The model under review builds one solid part; all positions refer to its coordinate system, in mm. A direction names the side the tool comes from. Round coordinates to 2 decimals unless told otherwise and drop trailing zeros. Write each loop counter-clockwise with the first axis right and the second up, starting at its lowest first coordinate (ties: lowest second). Pieces come first, ordered by that corner, then holes. Notation, with made-up numbers: (46, -34.5) -> (51, -34.5) arc R26 cw to (51, 2.5) -> close; hole circle Ø1 at (-27, -32.75). An arc over 180 degrees is marked (long way). Return JSON: item names as keys, results as strings. Group by question number.
1. Take a section at C-C, the plane z = 0.5. Write out the cut boundary in (x, y), then the cut area to 3 significant figures.
2. For line 1 along X through (y, z) = (-0.75, -2.25); line 2 along Z through (x, y) = (-3, -1.05); line 3 along X through (y, z) = (-0.4, 4.5), list the stretches that pass through material, from the lowest coordinate up. Write a range as from..to.
3. Take a section at D-D, the plane x = -2.25. Write out the cut boundary in (y, z), then the cut area to 3 significant figures.
4. Mouldability with a two-part tool opening along Z and no side actions: class faces 1 (the flat face through (-0.1, -2, -1.6)), 2 (the cylindrical face through (-5.79, -0.99, 0.75)), 3 (the cylindrical face through (-1.63, -0.99, -7.32)) as pulls with the +Z half, pulls with the -Z half, needs draft (parallel to the pull), parting line crosses it, or undercut.
5. Tool access review of faces 4 (the flat face through (-4.144, -0.986, -1.81)), 5 (the flat face through (-0.1, 0, -1.6)): name each direction out of +Z, -Z, +X, -X, +Y, -Y from which nothing blocks a thin tool from reaching the whole face with its end or side.
6. Take a section at B-B, the plane x = -0.5. Write out the cut boundary in (y, z).
7. Take a section at A-A, the plane y = -1.2. Write out the cut boundary in (x, z) (1 decimal), then the cut area to 3 significant figures.
from build123d import *

# Parameters (mm, degrees)
F1_DEPTH = 2


# Not quite as in the source:
# - ends of sketch curves that miss each other by under 0.0002 mm in the source are joined


with BuildPart() as f1:
    # F0 (on Front) → F1 (new body)
    with BuildSketch(Plane.XZ):
        with BuildLine():
            ThreePointArc((-7.5, 0), (0, -7.5), (7.5, 0))
            ThreePointArc((7.5, 0), (0, 7.5), (-7.5, 0))
        make_face()
        with BuildLine():
            ThreePointArc((-9.252e-06, -5.837642026), (-0.8154481123, -5.781304427), (-1.6149720231, -5.6113751006))
            Line((-1.6149720231, -5.6113751006), (0, -2.0297722424))
            Line((0, -2.0297722424), (1.6130763481, -5.6119564271))
            ThreePointArc((1.6130763481, -5.6119564271), (0.8143893667, -5.7809478456), (-9.252e-06, -5.837642026))
        make_face(mode=Mode.SUBTRACT)
        with BuildLine():
            ThreePointArc((-5.8376432623, 4.535e-07), (-5.7885795806, 0.7619262356), (-5.6402209677, 1.5108774116))
            Line((-5.6402209677, 1.5108774116), (-2.6057938378, -5.2253115461))
            ThreePointArc((-2.6057938378, -5.2253115461), (-4.9642649621, -3.0719201723), (-5.8376432623, 4.535e-07))
        make_face(mode=Mode.SUBTRACT)
        with BuildLine():
            ThreePointArc((5.8375074432, 8.164e-07), (4.9638082552, -3.0717207498), (2.6056583249, -5.2253113695))
            Line((2.6056583249, -5.2253113695), (5.6435948014, 1.498042557))
            ThreePointArc((5.6435948014, 1.498042557), (5.7887533107, 0.7552604254), (5.8375074432, 8.164e-07))
        make_face(mode=Mode.SUBTRACT)
        with BuildLine():
            Line((0, 1.9682461262), (-1.6421023797, 5.6034935248))
            ThreePointArc((-1.6421023797, 5.6034935248), (-0.8294183969, 5.7791792496), (-8.9799e-06, 5.8374974962))
            ThreePointArc((-8.9799e-06, 5.8374974962), (0.8283723862, 5.7788128003), (1.6402065238, 5.6039289974))
            Line((1.6402065238, 5.6039289974), (0, 1.9682461262))
        make_face(mode=Mode.SUBTRACT)
        with BuildLine():
            Line((0.990821727, 0.1571487487), (3.1334508081, 4.9261166556))
            ThreePointArc((3.1334508081, 4.9261166556), (3.9933572695, 4.2579147754), (4.7150061526, 3.4423429304))
            Line((4.7150061526, 3.4423429304), (2.0229239131, -2.5149786417))
            Line((2.0229239131, -2.5149786417), (0.9841275984, -0.2051414777))
            Line((0.9841275984, -0.2051414777), (-0.9841094572, -0.2051414777))
            Line((-0.9841094572, -0.2051414777), (-2.0228967012, -2.5149786417))
            Line((-2.0228967012, -2.5149786417), (-4.7110881859, 3.447911577))
            ThreePointArc((-4.7110881859, 3.447911577), (-3.9911114988, 4.2602728506), (-3.1337140349, 4.925981317))
            Line((-3.1337140349, 4.925981317), (-0.9841094572, 0.1571487487))
            Line((-0.9841094572, 0.1571487487), (0.990821727, 0.1571487487))
        make_face(mode=Mode.SUBTRACT)
    extrude(amount=F1_DEPTH)


solid = f1.part
Output:
{
 "1": {"outline": "(-7.48, -2) -> (-5.82, -2) -> (-5.82, 0) -> (-7.48, 0) -> close; (-5.18, -2) -> (-3.38, -2) -> (-3.38, 0) -> (-5.18, 0) -> close; (-1.14, -2) -> (1.14, -2) -> (1.14, 0) -> (-1.14, 0) -> close; (3.39, -2) -> (5.19, -2) -> (5.19, 0) -> (3.39, 0) -> close; (5.82, -2) -> (7.48, -2) -> (7.48, 0) -> (5.82, 0) -> close", "area": "18.5 mm^2"},
 "2": {"line 1": "x = -7.15..-5.39, -3.95..-2.14, -1.9..-0.1, 0.1..1.9, 2.14..3.95, 5.39..7.15", "line 2": "z = -6.87..-5.01, -4.35..-0.35, 4.63..6.87", "line 3": "x = -6..-3.72, -2.94..-1.14, 1.14..2.94, 3.72..6"},
 "3": {"outline": "(-2, -7.15) -> (0, -7.15) -> (0, -2.01) -> (-2, -2.01) -> close; (-2, 2.97) -> (0, 2.97) -> (0, 7.15) -> (-2, 7.15) -> close", "area": "18.7 mm^2"},
 "4": {"face 1": "needs draft", "face 2": "undercut", "face 3": "parting line crosses it"},
 "5": {"face 4": "+Y, -Y", "face 5": "+Z, -Z, +X, -X, +Y"},
 "6": {"outline": "(-2, -7.48) -> (0, -7.48) -> (0, -5.82) -> (-2, -5.82) -> close; (-2, -3.14) -> (0, -3.14) -> (0, -0.21) -> (-2, -0.21) -> close; (-2, 0.16) -> (0, 0.16) -> (0, 3.08) -> (-2, 3.08) -> close; (-2, 5.82) -> (0, 5.82) -> (0, 7.48) -> (-2, 7.48) -> close"},
 "7": {"outline": "circle Ø15 at (0, 0); hole (-5.8, 0) arc R5.8 ccw to (-2.6, -5.2) -> (-5.6, 1.5) arc R5.8 ccw to start; hole (-4.7, 3.4) -> (-2, -2.5) -> (-1, -0.2) -> (1, -0.2) -> (2, -2.5) -> (4.7, 3.4) arc R5.9 ccw to (3.1, 4.9) -> (1, 0.2) -> (-1, 0.2) -> (-3.1, 4.9) arc R5.9 ccw to start; hole (-1.6, -5.6) arc R5.8 ccw to (0, -5.8) arc R5.9 ccw to (1.6, -5.6) -> (0, -2) -> close; hole (-1.6, 5.6) -> (0, 2) -> (1.6, 5.6) arc R5.9 ccw to (0, 5.8) arc R5.8 ccw to start; hole (2.6, -5.2) arc R5.8 ccw to (5.8, 0) arc R5.9 ccw to (5.6, 1.5) -> close", "area": "125 mm^2"}
}
